Source: CAD feature listing. Evaluate the final solid. Frame: model axes, mm. Face numbers are marked on the shaded views. A direction names the side the tool comes from. Round coordinates to 2 decimals unless told otherwise and drop trailing zeros. Loops run counter-clockwise (first coordinate to the right, second up) from the corner with the lowest first, then second, coordinate; pieces in that order, holes last.
(1) Section D-D, the plane z = -31. Count the separate pieces of the cut face and the enclosed holes in it, plus the area to 3 significant figures.
(2) Material intervals for probe 1 along Y at (x, z) = (0, 5); probe 2 along Z at (x, y) = (-6, -32.5); probe 3 along X at (y, z) = (-52, -0.5), sorted ascending.
(3) First-contact query: pin 1 Ø12 at (x, y) = (-37.5, -38) entering from -Z; pin 2 Ø2 at (x, y) = (-6, -41.5) entering from +Z; pin 3 Ø17.5 at (y, z) = (-92.5, -15.5) entering from -X; pin 4 Ø12 at (y, z) = (-83.5, -3) entering from -X. Flat tips, straight axial feed; report the tip coordinate or a pass-through.
(4) Section A-A, the plane x = 0. Return the cut outline in (y, z), plus the area to 3 significant figures.
(5) Section C-C, the plane y = 40. Return the cut outline in (x, z), plus the area to 3 significant figures.
(6) Set-up query: the marked faces 1, 2, 3 and 4. Return all of +Z, -Z, +X, -X, +Y, -Y with unobstructed straight access to the full face (end or side cutting, diameter ignored); none if empty.
(7) Section B-B, the plane x = 40. Return the cut outline in (y, z).
```python
from build123d import *

# Parameters (mm, degrees)
F0_W     = 100
F0_H     = 100
F0_R     = 5
F0_R_2   = 25
F1_DEPTH = 15
F0_R_3   = 19.999999553
F2_DEPTH = 20
F3_DEPTH = 45
F5_W     = 15
F5_H     = 15
F10_R    = 1
F11_R    = 0.5


with BuildPart() as f1:
    # F0 (on Top) → F1 (new body)
    with BuildSketch(Plane.XY):
        Rectangle(F0_W, F0_H)
        with Locations((-40, 40)):
            Circle(F0_R, mode=Mode.SUBTRACT)
        Circle(F0_R_2, mode=Mode.SUBTRACT)
        with Locations((40, 40)):
            Circle(F0_R, mode=Mode.SUBTRACT)
        with Locations((40, 40)):
            Circle(F0_R)
        with Locations((-40, 40)):
            Circle(F0_R)
    extrude(amount=F1_DEPTH)

    # F0 (on Top) → F2 (join)
    with BuildSketch(Plane.XY):
        Circle(F0_R_2)
        Circle(F0_R_3, mode=Mode.SUBTRACT)
    extrude(amount=F2_DEPTH)

    # F0 (on Top) → F3 (join)
    with BuildSketch(Plane.XY):
        with Locations((-40, 40)):
            Circle(F0_R)
        with Locations((40, 40)):
            Circle(F0_R)
    extrude(amount=-F3_DEPTH)

    # F8: sweep along a path in F7
    with BuildLine(Plane.YZ.offset(50)) as f8_path:
        Line((-110, -45), (-50, 15))
    # F5 (on offset) → F8 (sweep)
    with BuildSketch(Plane.XY.offset(-45)):
        with Locations((42.5, -102.5)):
            Rectangle(F5_W, F5_H)
    sweep(path=f8_path.line)

    # F9: F1 across plane


with BuildPart() as f1_1:
    add(f1.part)
    add(f1.part.mirror(Plane.YZ))

    # F10
    f10_edges = [f1_1.edges().sort_by_distance(p)[0] for p in [
        (-35, -50, 7.5),
        (35, -50, 7.5),
        (-20, 0, 0),
        (20, 0, 10),
        (-20, 0, 20),
    ]]
    fillet(f10_edges, radius=F10_R)

    # F11
    f11_edges = [f1_1.edges().sort_by_distance(p)[0] for p in [
        (-25, 0, 20),
        (50, 0, 15),
        (0, 50, 15),
        (50, 50, 7.5),
        (-50, 50, 7.5),
        (-50, 0, 15),
        (-50, 0, 0),
        (0, 50, 0),
        (50, 0, 0),
        (50, -72.5, -22.5),
        (50, -80, -15),
        (-50, -80, -15),
        (-50, -72.5, -22.5),
        (-50, -102.5, -45),
        (-42.5, -95, -45),
        (-42.5, -110, -45),
        (35, -102.5, -45),
        (42.5, -110, -45),
        (-35, -102.5, -45),
        (50, -102.5, -45),
    ]]
    fillet(f11_edges, radius=F11_R)


solid = f1_1.part
```
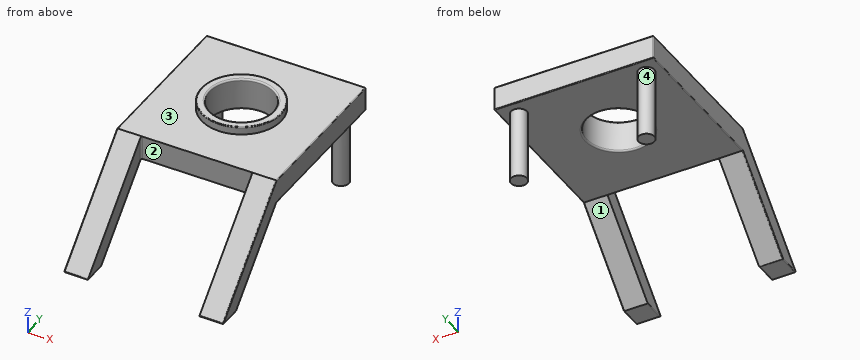
Output values:
1. separate pieces: 4
1. enclosed holes: 0
1. area: 607 mm2
2. probe 1: y = -50 to -20, 20 to 50
2. probe 2: z = 0 to 15
2. probe 3: x = -50 to -35, 35 to 50
3. pin 1: stops at z = 0
3. pin 2: stops at z = 15
3. pin 3: stops at x = -49.94
3. pin 4: passes through
4. outline: (-50, 0) - (-21, 0) arc R1 ccw to (-20, 1) - (-20, 19) arc R1 ccw to (-21, 20) - (-24.5, 20) arc R0.5 ccw to (-25, 19.5) - (-25, 15) - (-50, 15) - close; (20, 1) arc R1 ccw to (21, 0) - (49.5, 0) arc R0.5 ccw to (50, 0.5) - (50, 14.5) arc R0.5 ccw to (49.5, 15) - (25, 15) - (25, 19.5) arc R0.5 ccw to (24.5, 20) - (21, 20) arc R1 ccw to (20, 19) - close
4. area: 949 mm2
5. outline: (-50, 0.5) arc R0.5 ccw to (-49.5, 0) - (-45, 0) - (-45, -45) - (-35, -45) - (-35, 0) - (35, 0) - (35, -45) - (45, -45) - (45, 0) - (49.5, 0) arc R0.5 ccw to (50, 0.5) - (50, 14.5) arc R0.5 ccw to (49.5, 15) - (-49.5, 15) arc R0.5 ccw to (-50, 14.5) - close
5. area: 2,400 mm2
6. face 1: -Z, +X, -X
6. face 2: +Z, -Z, -Y
6. face 3: +Z
6. face 4: -Z
7. outline: (-109.15, -44.15) arc R0.5 ccw to (-108.79, -45) - (-95, -45) - (-50, 0) - (35, 0) - (35, -45) - (45, -45) - (45, 0) - (49.5, 0) arc R0.5 ccw to (50, 0.5) - (50, 14.5) arc R0.5 ccw to (49.5, 15) - (-50, 15) - close
